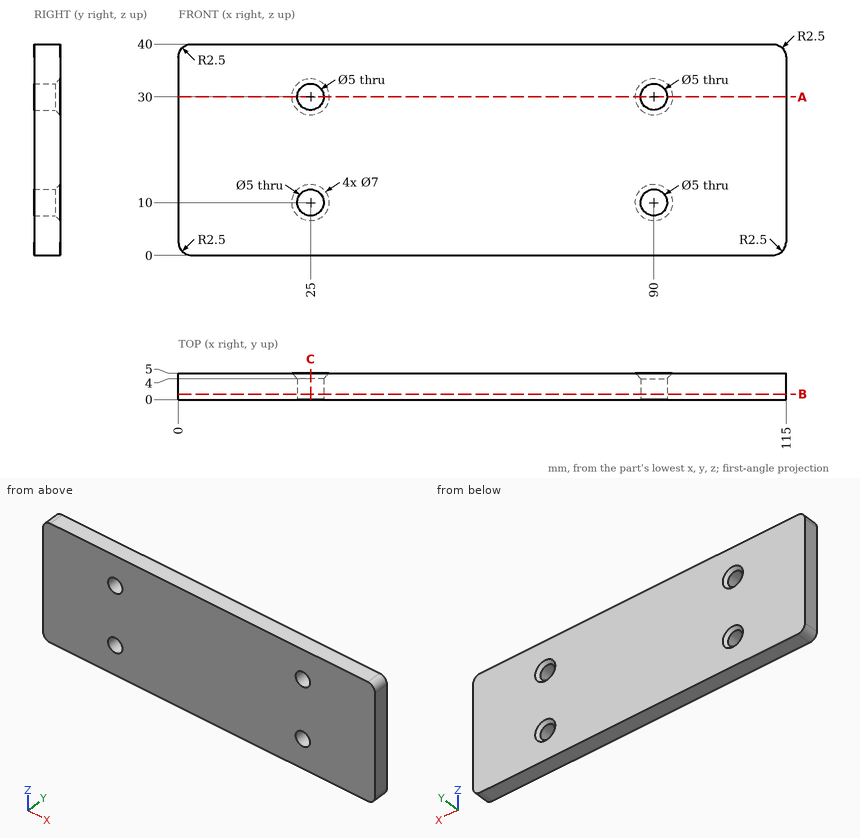
Geometry check sheet. Reference: drawing and pictorial views, mm from the part's lowest x, y, z. Give positions to 0.01 mm unless a question says otherwise; leave off trailing zeros. Loops run counter-clockwise (first coordinate to the right, second up) from the corner with the lowest first, then second, coordinate; pieces in that order, holes last. Notation, with made-up numbers: (32, 65.25) -> (71, 65.25) arc R14 ccw to (71, 71.25) -> close; hole circle Ø4 at (-31, 39.5). An arc over 180 degrees is marked (long way). Answer in a Markdown table with one row per item. Add a question column.
1) Gauge pin test, flat ends, axial feed: P1, Ø4.5, axis at x = 25, z = 10, coming from the -Y side; P2, Ø6.5, axis at x = 90, z = 30, coming from the +Y side. Record the tip position at first contact, or that the pin passes through.
2) Material ranges on probe 1 along X at (y, z) = (1.35, 30); probe 2 along Z at (x, y) = (90, 2.45); probe 3 along Z at (x, y) = (88, 3.45), recorded low to high. Write a range as from..to.
3) Cross-section at A-A on z = 30. Record the boundary of the cut face in (x, y).
4) Cross-section at B-B on y = 1.05. Record the boundary of the cut face in (x, z), and give its area (3 significant figures).
5) Cross-section at C-C on x = 25. Record the boundary of the cut face in (y, z).
Outcome:
| question | item | result |
|---|---|---|
| 1 | P1 | passes through |
| 1 | P2 | stops at y = 4.75 |
| 2 | probe 1 | x = 0..22.5, 27.5..87.5, 92.5..115 |
| 2 | probe 2 | z = 0..7.5, 12.5..27.5, 32.5..40 |
| 2 | probe 3 | z = 0..8.5, 11.5..28.5, 31.5..40 |
| 3 | outline | (0, 0) -> (22.5, 0) -> (22.5, 4) -> (21.5, 5) -> (0, 5) -> close; (27.5, 0) -> (87.5, 0) -> (87.5, 4) -> (86.5, 5) -> (28.5, 5) -> (27.5, 4) -> close; (92.5, 0) -> (115, 0) -> (115, 5) -> (93.5, 5) -> (92.5, 4) -> close |
| 4 | outline | (0, 2.5) arc R2.5 ccw to (2.5, 0) -> (112.5, 0) arc R2.5 ccw to (115, 2.5) -> (115, 37.5) arc R2.5 ccw to (112.5, 40) -> (2.5, 40) arc R2.5 ccw to (0, 37.5) -> close; hole circle Ø5 at (25, 10); hole circle Ø5 at (25, 30); hole circle Ø5 at (90, 10); hole circle Ø5 at (90, 30) |
| 4 | area | 4,520 mm^2 |
| 5 | outline | (0, 0) -> (5, 0) -> (5, 6.5) -> (4, 7.5) -> (0, 7.5) -> close; (0, 12.5) -> (4, 12.5) -> (5, 13.5) -> (5, 26.5) -> (4, 27.5) -> (0, 27.5) -> close; (0, 32.5) -> (4, 32.5) -> (5, 33.5) -> (5, 40) -> (0, 40) -> close |
